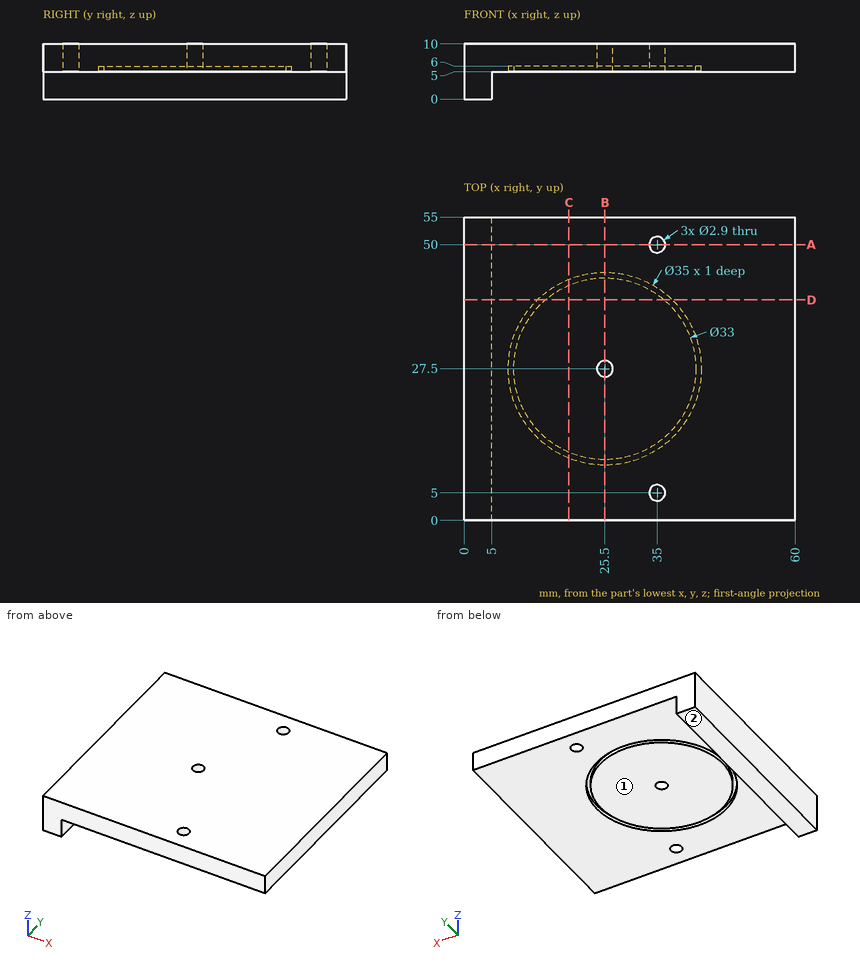
Answer from the drawing. Dimensions are ordinates in mm from the lowest x, y and z of the part. A direction names the side the tool comes from. Coordinates: 2 decimals unless noted, no trailing zeros. Write each loop counter-clockwise with the first axis right and the second up, starting at its lowest first coordinate (ties: lowest second). Pieces come first, ordered by that corner, then holes. Notation, with made-up numbers: (-19, 59.25) - (36, 59.25) arc R25 cw to (36, 90.25) - close; hole circle Ø4 at (-29, 28). An arc over 180 degrees is marked (long way). Answer as CSV lines item,"result".
1. A tool of negligible diameter and unlimited length cuts with its end or side. For the marked faces 1 and 2, from which of +Z, -Z, +X, -X, +Y, -Y can it reach the whole face along a straight path? Write none if from no direction.
Computed values:
face 1,"-Z, +X, +Y, -Y"
face 2,"-Z, +X, -X, +Y, -Y"
2. Find section B-B (x = 25.5). Give the vertices of the cut face in (y, z), plus the area to 4 significant figures.
Computed values:
outline,"(0, 5) - (10, 5) - (10, 6) - (11, 6) - (11, 5) - (26.05, 5) - (26.05, 10) - (0, 10) - close; (28.95, 5) - (44, 5) - (44, 6) - (45, 6) - (45, 5) - (55, 5) - (55, 10) - (28.95, 10) - close"
area,"258.5 mm²"
3. Straight lines are drawn through the part: line 1 (Y direction, x = 35, z = 7.15); line 2 (Y direction, x = 25.5, z = 5.65); line 3 (X direction, y = 50, z = 7). For each, find the intervals that lie inside material, in ascending order. Write a range as [from, to].
Computed values:
line 1,"y = [0, 3.55], [6.45, 48.55], [51.45, 55]"
line 2,"y = [0, 10], [11, 26.05], [28.95, 44], [45, 55]"
line 3,"x = [0, 33.55], [36.45, 60]"
4. Find section D-D (y = 40). Give the vertices of the cut face in (x, z).
Computed values:
outline,"(0, 0) - (5, 0) - (5, 5) - (13.25, 5) - (13.25, 6) - (14.73, 6) - (14.73, 5) - (36.27, 5) - (36.27, 6) - (37.75, 6) - (37.75, 5) - (60, 5) - (60, 10) - (0, 10) - close"
5. Find section C-C (x = 19). Give the vertices of the cut face in (y, z), plus the area to 3 significant figures.
Computed values:
outline,"(0, 5) - (11.25, 5) - (11.25, 6) - (12.33, 6) - (12.33, 5) - (42.67, 5) - (42.67, 6) - (43.75, 6) - (43.75, 5) - (55, 5) - (55, 10) - (0, 10) - close"
area,"273 mm²"
6. Find section A-A (y = 50). Give the vertices of the cut face in (x, z), plus the area to 4 significant figures.
Computed values:
outline,"(0, 0) - (5, 0) - (5, 5) - (33.55, 5) - (33.55, 10) - (0, 10) - close; (36.45, 5) - (60, 5) - (60, 10) - (36.45, 10) - close"
area,"310.5 mm²"
7. Given P1, Ø1.5, axis at x = 12.5, y = 27, coming from the -Z side; P2, Ø1, axis at y = 15, z = 3, coming from the +X side, each flat-ended and moving along its own axis, determine where each tip first touches the part or whether it passes through.
Computed values:
P1,"stops at z = 5"
P2,"stops at x = 5"
